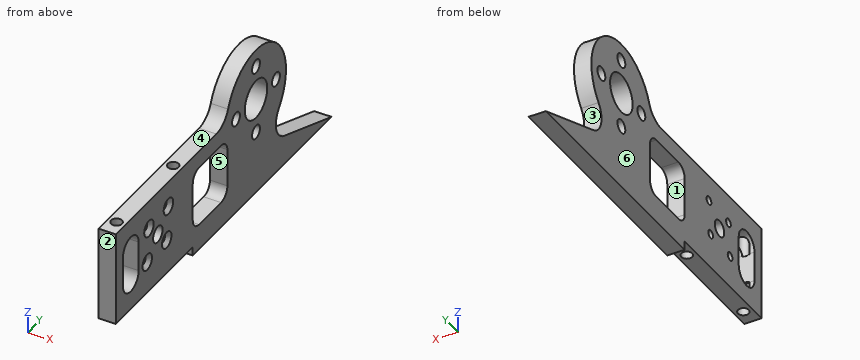
```python
from build123d import *

# Parameters (mm, degrees)
F0_R           = 3
F0_R_2         = 2.5
F0_R_3         = 7.14375
F1_DEPTH       = 6.35
F3_D           = 3
F3_CSINK_D     = 6
F3_CSINK_ANGLE = 90
F5_DEPTH       = 25
F6_W           = 6.35
F6_H           = 38
F7_DEPTH       = 37.876
F9_D           = 4
F9_DEPTH       = 12
F9_TIP         = 1.2017212381
F11_D          = 4
F11_DEPTH      = 12
F11_TIP        = 1.2017212381


with BuildPart() as f1:
    # F0 (on Right) → F1 (new body)
    with BuildSketch(Plane.YZ):
        with BuildLine():
            ThreePointArc((17.8751346366, -25.0354456965), (12.8773903734, -19.5640491806), (14.5155336292, -12.3370086917))
            ThreePointArc((14.5155336292, -12.3370086917), (9.7791608288, 16.348410121), (-17.735210007, 6.9544824399))
            ThreePointArc((-17.735210007, 6.9544824399), (-20.675525796, 3.2657587243), (-25.1830672278, 1.875))
            Line((-25.1830672278, 1.875), (-127.0762324528, 1.875))
            Line((-127.0762324528, 1.875), (-127.0762324528, -4.475))
            Line((-127.0762324528, -4.475), (-93.0762324528, -4.475))
            ThreePointArc((-93.0762324528, -4.475), (-90.247805328, -5.6465728753), (-89.0762324528, -8.475))
            Line((-89.0762324528, -8.475), (-89.0762324528, -22.475))
            ThreePointArc((-89.0762324528, -22.475), (-90.247805328, -25.3034271247), (-93.0762324528, -26.475))
            Line((-93.0762324528, -26.475), (-127.0762324528, -26.475))
            Line((-127.0762324528, -26.475), (-127.0762324528, -32.825))
            Line((-127.0762324528, -32.825), (-40.201, -32.825))
            Line((-40.201, -32.825), (-40.201, -36))
            Line((-40.201, -36), (48, -36))
            Line((48, -36), (17.8751346366, -25.0354456965))
        make_face()
        with Locations((-62.3762324528, -14.325)):
            Circle(F0_R, mode=Mode.SUBTRACT)
        with BuildLine():
            ThreePointArc((-40.201, -8.475), (-39.0294271247, -5.6465728753), (-36.201, -4.475))
            Line((-36.201, -4.475), (-22.201, -4.475))
            ThreePointArc((-22.201, -4.475), (-19.3725728753, -5.6465728753), (-18.201, -8.475))
            Line((-18.201, -8.475), (-18.201, -22.475))
            ThreePointArc((-18.201, -22.475), (-19.3725728753, -25.3034271247), (-22.201, -26.475))
            Line((-22.201, -26.475), (-36.201, -26.475))
            ThreePointArc((-36.201, -26.475), (-39.0294271247, -25.3034271247), (-40.201, -22.475))
            Line((-40.201, -22.475), (-40.201, -8.475))
        make_face(mode=Mode.SUBTRACT)
        with Locations((0, -12.7)):
            Circle(F0_R_2, mode=Mode.SUBTRACT)
        with Locations((-12.7, 0)):
            Circle(F0_R_2, mode=Mode.SUBTRACT)
        Circle(F0_R_3, mode=Mode.SUBTRACT)
        with Locations((12.7, 0)):
            Circle(F0_R_2, mode=Mode.SUBTRACT)
        with Locations((0, 12.7)):
            Circle(F0_R_2, mode=Mode.SUBTRACT)
    extrude(amount=F1_DEPTH)

    # F3 (through all)
    with Locations(Plane.YZ.offset(6.35)):
        with Locations((-55.6587180315, -7.6074855787), (-68.0330867022, -8.6681457505), (-69.093746874, -21.0425144213), (-56.7193782033, -19.9818542495)):
            CounterSinkHole(F3_D / 2, F3_CSINK_D / 2, counter_sink_angle=F3_CSINK_ANGLE)

    # F4 (on face) → F5 (cut)
    with BuildSketch(Plane.YZ.offset(6.35)):
        with BuildLine():
            ThreePointArc((-74.5762324528, -9.975), (-79.5762324528, -4.975), (-84.5762324528, -9.975))
            Line((-84.5762324528, -9.975), (-84.5762324528, -20.975))
            ThreePointArc((-84.5762324528, -20.975), (-79.5762324528, -25.975), (-74.5762324528, -20.975))
            Line((-74.5762324528, -20.975), (-74.5762324528, -9.975))
        make_face()
    extrude(amount=-F5_DEPTH, mode=Mode.SUBTRACT)

    # F6 (on face) → F7 (cut, through all)
    with BuildSketch(Plane.XY.offset(1.875)):
        with Locations((3.175, -108.0762324528)):
            Rectangle(F6_W, F6_H)
    extrude(amount=-F7_DEPTH, mode=Mode.SUBTRACT)

    # F9
    with Locations(Plane.XY.offset(1.875)):
        with Locations((3.175, -47.0762324528), (3.175, -83.0762324528)):
            Hole(F9_D / 2, depth=F9_DEPTH)
            with Locations((0, 0, -(F9_DEPTH + F9_TIP / 2))):  # 118° drill point
                Cone(0, F9_D / 2, F9_TIP, mode=Mode.SUBTRACT)

    # F11
    with Locations(Plane(origin=(0, 0, -32.825), x_dir=(1, 0, 0), z_dir=(0, 0, -1))):
        with Locations((3.175, 47.0762324528), (3.175, 83.0762324528)):
            Hole(F11_D / 2, depth=F11_DEPTH)
            with Locations((0, 0, -(F11_DEPTH + F11_TIP / 2))):  # 118° drill point
                Cone(0, F11_D / 2, F11_TIP, mode=Mode.SUBTRACT)


solid = f1.part
```
Could you check a few things on this model? Use its own coordinates, in mm. Face numbers are marked on the shaded views. A direction names the side the tool comes from. Give positions to 0.01 mm unless a question says otherwise; leave off trailing zeros. Write each loop counter-clockwise with the first axis right and the second up, starting at its lowest first coordinate (ties: lowest second). Pieces come first, ordered by that corner, then holes. Notation, with made-up numbers: (37.5, -1) - (55.5, -1) arc R11 cw to (55.5, 10) - close; hole circle Ø11 at (38, 54.5). An arc over 180 degrees is marked (long way). One line per item, written item: value. Start each with the question number.
Item 1: Imagine slicing it at B-B, the plane y = 0. List the corners of the cut face in (x, z) for me.
Item 2: If we mould it in two halves opening along Y, with no side actions, what happens to the marked faces 1, 2 and 3? For each: +Y half, -Y half, draft (parallel to the pull), parting line (faces both ways), or undercut.
Item 3: I'm going to push flat-ended pins straight in: pin 1 (1.5 mm diameter, centred on x = 5.5, z = -22.5, fed in from +Y); pin 2 (1.9 mm diameter, centred on x = 3.5, z = -17.5, fed in from +Y); pin 3 (4 mm diameter, centred on y = -68.03, z = -8.67, fed in from +X). Where does each tip first touch, or does it pass through?
Item 4: Imagine slicing it at D-D, the plane z = 12.7. List the corners of the cut face in (x, y) for me, and give its area (3 significant figures).
Item 5: Imagine slicing it at C-C, the plane z = 0. List the corners of the cut face in (x, y) for me (3 decimals), and give its area (3 significant figures).
Item 6: Please list where these lines run through material, in increasing order: line 1 (Z direction, x = 0.5, y = -34.5) (3 decimals); line 2 (Y direction, x = 4.5, z = -8.5); line 3 (Y direction, x = 6, z = -24). Write a range as from..to.
Item 7: Which directions (+Z, -Z, +X, -X, +Y, -Y) give clear straight access to the entire face, cutting with the end or side of a thin tool? Please do the marked faces 4, 5 and 6.
Item 8: Imagine slicing it at A-A, the plane y = -32. List the corners of the cut face in (x, z) for me (3 decimals), and give its area (3 significant figures).
Geometry says:
1. outline: (0, -36) - (6.35, -36) - (6.35, -15.2) - (0, -15.2) - close; (0, -10.2) - (6.35, -10.2) - (6.35, -7.14) - (0, -7.14) - close; (0, 7.14) - (6.35, 7.14) - (6.35, 10.2) - (0, 10.2) - close; (0, 15.2) - (6.35, 15.2) - (6.35, 19.05) - (0, 19.05) - close
2. face 1: undercut
2. face 2: -Y half
2. face 3: +Y half
3. pin 1: y = 15.03
3. pin 2: y = 12.67
3. pin 3: x = 5.35
4. outline: (0, -14.2) - (6.35, -14.2) - (6.35, -2.5) - (0, -2.5) - close; (0, 2.5) - (6.35, 2.5) - (6.35, 14.2) - (0, 14.2) - close
4. area: 149 mm^2
5. outline: (0, -89.076) - (6.35, -89.076) - (6.35, -15.2) - (0, -15.2) - close; (0, -10.2) - (6.35, -10.2) - (6.35, -7.144) - (0, -7.144) - close; (0, 7.144) - (6.35, 7.144) - (6.35, 10.2) - (0, 10.2) - close; (0, 15.2) - (6.35, 15.2) - (6.35, 19.05) - (0, 19.05) - close; hole circle Ø4 at (3.175, -83.076); hole circle Ø4 at (3.175, -47.076)
5. area: 507 mm^2
6. line 1: -36..-26.475, -4.475..1.875
6. line 2: -89.08..-84.57, -74.8..-69.52, -66.54..-56.86, -54.45..-48.57, -45.58..-40.2, -18.2..17.05
6. line 3: -89.08..-83.56, -75.6..-39.9, -18.5..15.92
7. face 4: +Z, +X, -X, -Y
7. face 5: +X, -X
7. face 6: +Z, -Z, -X, +Y, -Y
8. outline: (0, -36) - (6.35, -36) - (6.35, -26.475) - (0, -26.475) - close; (0, -4.475) - (6.35, -4.475) - (6.35, 1.875) - (0, 1.875) - close
8. area: 101 mm^2
